Can you work these out from the model? Positions are in its coordinate system, mm. A direction names the side the tool comes from. Coordinates: 2 decimals unless noted, no trailing zeros. Write each loop counter-clockwise with the first axis right and the second up, starting at its lowest first coordinate (ties: lowest second). Pieces come first, ordered by that corner, then holes. Notation, with made-up numbers: (18.25, -8) - (42.25, -8) arc R16 ccw to (42.25, -1) - close; hole circle Ø7 at (70, 37). An arc over 180 degrees is marked (long way). Use one line per item in the form item = value. Start each with the question number.
(1) If we section it at A-A on z = -49: Please give me the cut outline in (x, y), then the cut area to 3 significant figures.
(2) Thinking about a two-plate mould opening in Y: for faces 1 (the face through (-57.5, -3, 32)), 2 (the face through (61, -2.5, 32)), 3 (the face through (62.007, -3.512, 72.316)), 4 (the face through (-61, -3.5, 32)), which applies, pulls with the +Y half, pulls with the -Y half, needs draft (parallel to the pull), parting line crosses it, or undercut?
(3) For pin 1 Ø0.6 at (x, y) = (19.5, -0.5) entering from +Z (3 decimals); pin 2 Ø1.5 at (x, z) = (28.5, 3.5) entering from -Y; pin 3 Ø2.5 at (x, z) = (-60.5, 30) entering from -Y, each with a flat end and sliding along its axis, tell me the tip position at first contact or that it passes through.
(4) On a 3-axis mill with a long thin cutter (end or side, diameter ignored), from which of +Z, -Z, +X, -X, +Y, -Y can I reach the whole of each face in a straight line? I mean faces 5 (the face through (-57.5, -3, -41)), 6 (the face through (61, -3.5, 32)), 7 (the face through (-61.5, -4, 74)), 8 (the face through (61, -2.5, -41)). Say none if no direction works.
(5) If I drill on probe 1 along X at (y, z) = (-4.5, 65); probe 2 along Y at (x, z) = (1, 17), over which ranges is the centre line in solid material (lowest first)? Write a range as from..to.
(6) If we section it at B-B on x = 37: Please give me the cut outline in (y, z) (3 decimals), then the cut area to 3 significant figures.
```python
from build123d import *

# Parameters (mm, degrees)
F0_W      = 1.2
F0_H      = 131.87
F0_W_2    = 127.4
F1_DEPTH  = 8.5
F2_W      = 125
F2_H      = 131.87
F3_DEPTH  = 8
F4_W      = 2.4
F4_H      = 8.5
F5_DEPTH  = 12.9
F6_R      = 1.6
F7_DEPTH  = 1
F9_DEPTH  = 3
F10_W     = 125
F10_H     = 2
F11_DEPTH = 130


# Not quite as in the source:
# - a pattern or mirror of a feature is missing from the dataset's text; its kind, count and spacing are read off the source's solid


with BuildPart() as f1:
    # F0 (on Front) → F1 (new body)
    with BuildSketch(Plane.XZ):
        with Locations((-64.3, 0)):
            Rectangle(F0_W, F0_H)
        Rectangle(F0_W_2, F0_H)
        with Locations((64.3, 0)):
            Rectangle(F0_W, F0_H)
    extrude(amount=F1_DEPTH)

    # F2 (on face) → F3 (cut)
    with BuildSketch(Plane.XZ.offset(8.5)):
        Rectangle(F2_W, F2_H)
    extrude(amount=-F3_DEPTH, mode=Mode.SUBTRACT)

    # F4 (on face) → F5 (join)
    with BuildSketch(Plane.XY.offset(65.935)):
        with Locations((-63.7, -4.25)):
            Rectangle(F4_W, F4_H)
        with Locations((63.7, -4.25)):
            Rectangle(F4_W, F4_H)
    extrude(amount=F5_DEPTH)

    # F6 (on face) → F7 (join)
    with BuildSketch(Plane.YZ.offset(-62.5)):
        with Locations((-4.25, 73.735)):
            Circle(F6_R)
    f7 = extrude(amount=F7_DEPTH)

    # F7_copies: F7 across plane
    add(f7.mirror(Plane(origin=(0, 0, 0), x_dir=(0, 0, 1), z_dir=(1, 0, 0))))

    # F8 (on face) → F9 (join)
    with BuildSketch(Plane.XZ.offset(0.5)):
        with BuildLine():
            Line((-62.5, -35.935), (-62.5, -45.935))
            ThreePointArc((-62.5, -45.935), (-57.5, -40.935), (-62.5, -35.935))
        make_face()
        with BuildLine():
            Line((-62.5, 37.065), (-62.5, 27.065))
            ThreePointArc((-62.5, 27.065), (-57.5, 32.065), (-62.5, 37.065))
        make_face()
    f9 = extrude(amount=F9_DEPTH)

    # F9_copies: F9 across plane
    add(f9.mirror(Plane(origin=(0, 0, 0), x_dir=(0, 0, 1), z_dir=(1, 0, 0))))

    # F10 (on face) → F11 (cut)
    with BuildSketch(Plane(origin=(0, 0, -65.935), x_dir=(1, 0, 0), z_dir=(0, 0, -1))):
        with Locations((0, 1.5)):
            Rectangle(F10_W, F10_H)
    extrude(amount=-F11_DEPTH, mode=Mode.SUBTRACT)


solid = f1.part
```
Reported:
q1.outline = (-64.9, -8.5) - (-62.5, -8.5) - (-62.5, -0.5) - (62.5, -0.5) - (62.5, -8.5) - (64.9, -8.5) - (64.9, 0) - (-64.9, 0) - close
q1.area = 103 mm2
q2.face_1 = needs draft
q2.face_2 = undercut
q2.face_3 = parting line crosses it
q2.face_4 = pulls with the -Y half
q3.pin_1 = 65.935
q3.pin_2 = -0.5
q3.pin_3 = -3.5
q4.face_5 = -Y
q4.face_6 = -Z, -Y
q4.face_7 = +Z, +Y, -Y
q4.face_8 = +Z, -Z
q5.probe_1 = -64.9..-62.5, 62.5..64.9
q5.probe_2 = -0.5..0
q6.outline = (-0.5, -65.935) - (0, -65.935) - (0, 65.935) - (-0.5, 65.935) - close
q6.area = 65.9 mm2
